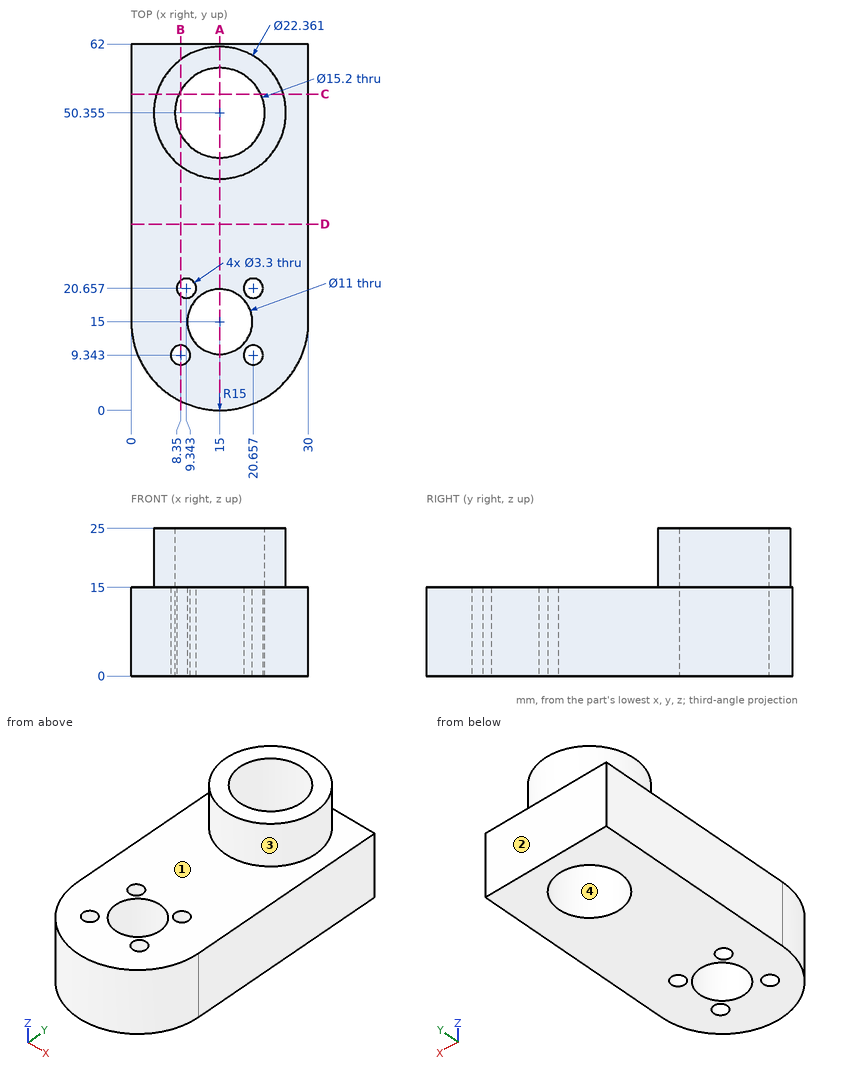
Can you work these out from the drawing? Everything is in mm from the part's minimum corner. Give positions to 0.01 mm unless a question says otherwise; leave off trailing zeros. Write each loop counter-clockwise with the first axis right and the second up, starting at its lowest first coordinate (ties: lowest second). Pieces come first, ordered by that corner, then holes. Notation, with made-up numbers: (32.5, -2.75) -> (80.5, -2.75) arc R14 cw to (80.5, 11.25) -> close; hole circle Ø7 at (63, 7.25). An arc over 180 degrees is marked (long way). Write each question's results on one line, items separated by ' | '. Start each with the question number.
Q1. Suppose I cut it at D-D, the plane y = 31.5. List the corners of the cut face in (x, z) for me, and give its area (3 significant figures).
Q2. We'd pull the mould along Y, two halves only. Please class the marked faces 1, 2, 3 and 4: +Y half, -Y half, draft (parallel to the pull), parting line (faces both ways), or undercut.
Q3. I need wall thicknesses on probe 1 along Y at (x, z) = (15, 11) (1 decimal); probe 2 along Y at (x, z) = (13.5, 7) (1 decimal); probe 3 along Y at (x, z) = (19.5, 3.5) (1 decimal). Which ranges of each line are inside material? Lowest first, please.
Q4. I'm going to push flat-ended pins straight in: pin 1 Ø10 at (x, y) = (15, 15) entering from -Z; pin 2 Ø4 at (y, z) = (40, 18.5) entering from -X; pin 3 Ø1 at (x, y) = (5.5, 19) entering from +Z; pin 4 Ø8 at (x, z) = (23.5, 9) entering from -Y. Where does each tip first touch, or does it pass through?
Q5. Suppose I cut it at B-B, the plane x = 8.35. List the corners of the cut face in (y, z) for me (1 decimal).
Q6. Suppose I cut it at A-A, the plane x = 15. List the corners of the cut face in (y, z) for me (1 decimal).
Q7. Suppose I cut it at C-C, the plane y = 53.5. List the corners of the cut face in (x, z) for me.
Outcome:
1) outline: (0, 0) -> (30, 0) -> (30, 15) -> (0, 15) -> close | area: 450 mm2
2) face 1: draft | face 2: +Y half | face 3: parting line | face 4: undercut
3) probe 1: 0 to 9.5, 20.5 to 42.8, 58 to 62 | probe 2: 0.1 to 9.7, 20.3 to 42.9, 57.8 to 62 | probe 3: 0.7 to 8.2, 10.5 to 11.8, 18.2 to 19.5, 21.8 to 44.2, 56.5 to 62
4) pin 1: through | pin 2: x = 7.57 | pin 3: z = 15 | pin 4: y = 0.69
5) outline: (1.6, 0) -> (7.7, 0) -> (7.7, 15) -> (1.6, 15) -> close; (11, 0) -> (19.3, 0) -> (19.3, 15) -> (11, 15) -> close; (22, 0) -> (46.7, 0) -> (46.7, 25) -> (41.4, 25) -> (41.4, 15) -> (22, 15) -> close; (54, 0) -> (62, 0) -> (62, 15) -> (59.3, 15) -> (59.3, 25) -> (54, 25) -> close
6) outline: (0, 0) -> (9.5, 0) -> (9.5, 15) -> (0, 15) -> close; (20.5, 0) -> (42.8, 0) -> (42.8, 25) -> (39.2, 25) -> (39.2, 15) -> (20.5, 15) -> close; (58, 0) -> (62, 0) -> (62, 15) -> (61.5, 15) -> (61.5, 25) -> (58, 25) -> close
7) outline: (0, 0) -> (8.08, 0) -> (8.08, 25) -> (4.27, 25) -> (4.27, 15) -> (0, 15) -> close; (21.92, 0) -> (30, 0) -> (30, 15) -> (25.73, 15) -> (25.73, 25) -> (21.92, 25) -> close
